from build123d import *

# Parameters (mm, degrees)
F1_DEPTH = 4.7625
F3_D     = 57.15
F4_D     = 25.4


with BuildPart() as f1:
    # F0 (on Front) → F1 (new body, symmetric)
    with BuildSketch(Plane.XZ):
        with BuildLine():
            ThreePointArc((63.5, 161.311665), (-6.276947, 224.500667), (-62.259053, 148.819256))
            ThreePointArc((-62.259053, 148.819256), (0, 161.317577), (62.259053, 148.819256))
            ThreePointArc((62.259053, 148.819256), (63.189002, 155.034718), (63.5, 161.311665))
        make_face()
        with BuildLine():
            ThreePointArc((-62.259053, 148.819256), (-51.584807, 124.281169), (-31.75, 106.319052))
            Line((-31.75, 106.319052), (0, 161.311665))
            Line((0, 161.311665), (31.75, 106.319052))
            ThreePointArc((31.75, 106.319052), (51.584807, 124.281169), (62.259053, 148.819256))
            ThreePointArc((62.259053, 148.819256), (0, 161.317577), (-62.259053, 148.819256))
        make_face()
        with BuildLine():
            ThreePointArc((-107.95, -25.663219), (-84.707387, -48.905833), (-76.2, -80.655833))
            Line((-76.2, -80.655833), (0, -80.655833))
            Line((0, -80.655833), (76.2, -80.655833))
            ThreePointArc((76.2, -80.655833), (84.707387, -48.905833), (107.95, -25.663219))
            Line((107.95, -25.663219), (69.849998, 40.327919))
            Line((69.849998, 40.327919), (31.75, 106.319052))
            ThreePointArc((31.75, 106.319052), (0, 97.811665), (-31.75, 106.319052))
            Line((-31.75, 106.319052), (-69.849998, 40.327919))
            Line((-69.849998, 40.327919), (-107.95, -25.663219))
        make_face()
        with BuildLine():
            Line((69.849998, 40.327919), (107.95, -25.663219))
            ThreePointArc((107.95, -25.663219), (133.423053, -17.466831), (160.010782, -20.491706))
            add(Edge.make_bspline(
                [(69.849998, 40.327919), (69.849999, 40.327918), (86.141954, 12.109423), (123.076369, -4.191142), (160.010782, -20.491706)],
                knots=[108.756574, 108.756574, 108.756574, 108.756574, 108.756578, 217.513155, 217.513155, 217.513155, 217.513155], degree=3))
        make_face()
        with BuildLine():
            ThreePointArc((-160.010782, -20.491706), (-133.423053, -17.466831), (-107.95, -25.663219))
            Line((-107.95, -25.663219), (-69.849998, 40.327919))
            add(Edge.make_bspline(
                [(-160.010782, -20.491706), (-123.076369, -4.191142), (-86.141954, 12.109423), (-69.849999, 40.327918), (-69.849998, 40.327919)],
                knots=[0, 0, 0, 0, 108.756578, 108.756581, 108.756581, 108.756581, 108.756581], degree=3))
        make_face()
        with BuildLine():
            Line((0, 161.311665), (-31.75, 106.319052))
            ThreePointArc((-31.75, 106.319052), (0, 97.811665), (31.75, 106.319052))
            Line((31.75, 106.319052), (0, 161.311665))
        make_face()
        with BuildLine():
            ThreePointArc((160.010782, -20.491706), (139.705119, -80.658788), (97.751729, -128.327549))
            ThreePointArc((97.751729, -128.327549), (165.858505, -138.517587), (203.2, -80.655833))
            ThreePointArc((203.2, -80.655833), (191.284807, -43.625336), (160.010782, -20.491706))
        make_face()
        with BuildLine():
            ThreePointArc((107.95, -25.663219), (84.707387, -48.905833), (76.2, -80.655833))
            Line((76.2, -80.655833), (139.7, -80.655833))
            Line((139.7, -80.655833), (107.95, -25.663219))
        make_face()
        with BuildLine():
            Line((139.7, -80.655833), (76.2, -80.655833))
            ThreePointArc((76.2, -80.655833), (81.838246, -106.814338), (97.751729, -128.327549))
            ThreePointArc((97.751729, -128.327549), (139.705119, -80.658788), (160.010782, -20.491706))
            ThreePointArc((160.010782, -20.491706), (133.423053, -17.466831), (107.95, -25.663219))
            Line((107.95, -25.663219), (139.7, -80.655833))
        make_face()
        with BuildLine():
            Line((31.75, 106.319052), (69.849998, 40.327919))
            add(Edge.make_bspline(
                [(62.259053, 148.819256), (57.908549, 108.682834), (53.558045, 68.546413), (69.849998, 40.327919)],
                knots=[0, 0, 0, 0, 108.756574, 108.756574, 108.756574, 108.756574], degree=3))
            ThreePointArc((62.259053, 148.819256), (51.584807, 124.281169), (31.75, 106.319052))
        make_face()
        with BuildLine():
            Line((0, -80.655833), (-76.2, -80.655833))
            ThreePointArc((-76.2, -80.655833), (-81.838246, -106.814338), (-97.751729, -128.327549))
            add(Edge.make_bspline(
                [(-97.751729, -128.327549), (-65.16782, -104.491691), (-32.58391, -80.655833), (0, -80.655833)],
                knots=[0, 0, 0, 0, 108.756578, 108.756578, 108.756578, 108.756578], degree=3))
        make_face()
        with BuildLine():
            Line((76.2, -80.655833), (0, -80.655833))
            add(Edge.make_bspline(
                [(0, -80.655833), (32.58391, -80.655833), (65.16782, -104.491691), (97.751729, -128.327549)],
                knots=[108.756578, 108.756578, 108.756578, 108.756578, 217.513155, 217.513155, 217.513155, 217.513155], degree=3))
            ThreePointArc((97.751729, -128.327549), (81.838246, -106.814338), (76.2, -80.655833))
        make_face()
        with BuildLine():
            ThreePointArc((-97.751729, -128.327549), (-81.838246, -106.814338), (-76.2, -80.655833))
            Line((-76.2, -80.655833), (-139.7, -80.655833))
            Line((-139.7, -80.655833), (-107.95, -25.663219))
            ThreePointArc((-107.95, -25.663219), (-133.423053, -17.466831), (-160.010782, -20.491706))
            ThreePointArc((-160.010782, -20.491706), (-139.705119, -80.658788), (-97.751729, -128.327549))
        make_face()
        with BuildLine():
            Line((-139.7, -80.655833), (-76.2, -80.655833))
            ThreePointArc((-76.2, -80.655833), (-84.707387, -48.905833), (-107.95, -25.663219))
            Line((-107.95, -25.663219), (-139.7, -80.655833))
        make_face()
        with BuildLine():
            ThreePointArc((-160.010782, -20.491706), (-194.692613, -112.405833), (-97.751729, -128.327549))
            ThreePointArc((-97.751729, -128.327549), (-139.705119, -80.658788), (-160.010782, -20.491706))
        make_face()
        with BuildLine():
            add(Edge.make_bspline(
                [(-69.849998, 40.327919), (-53.558045, 68.546413), (-57.908549, 108.682834), (-62.259053, 148.819256)],
                knots=[108.756581, 108.756581, 108.756581, 108.756581, 217.513155, 217.513155, 217.513155, 217.513155], degree=3))
            Line((-69.849998, 40.327919), (-31.75, 106.319052))
            ThreePointArc((-31.75, 106.319052), (-51.584807, 124.281169), (-62.259053, 148.819256))
        make_face()
    extrude(amount=F1_DEPTH, both=True)

    # F3 (through all)
    with Locations(Plane.XZ.offset(4.7625)):
        with Locations((-139.7, -80.655833), (139.7, -80.655833), (0, 161.311665)):
            Hole(F3_D / 2)

    # F4 (through all)
    with Locations(Plane.XZ.offset(4.7625)):
        with Locations((0, 0)):
            Hole(F4_D / 2)


solid = f1.part
Geometry check sheet. Reference: the model listing, model coordinates, mm. Round coordinates to 2 decimals unless told otherwise and drop trailing zeros. Write each loop counter-clockwise with the first axis right and the second up, starting at its lowest first coordinate (ties: lowest second). Pieces come first, ordered by that corner, then holes.
Item 1: Section check C-C (y = 3). Give the number of separate pieces and of enclosed holes in the cut face, plus the area to 3 significant figures.
Determined:
separate pieces: 1
enclosed holes: 4
area: 63,500 mm2
Item 2: Material ranges on line 1 along Z through (x, y) = (0, 1.75); line 2 along X through (y, z) = (2, -100); line 3 along X through (y, z) = (3, -106.5), recorded low to high.
Determined:
line 1: z = -80.66 to -12.7, 12.7 to 132.74, 189.89 to 224.81
line 2: x = -200.18 to -160.73, -118.67 to -56.6, 56.6 to 118.67, 160.73 to 200.18
line 3: x = -197.7 to -151.89, -127.51 to -66.89, 66.89 to 127.51, 151.89 to 197.7
Item 3: Section check A-A (z = -74.5). Record the boundary of the cut face in (x, y), plus the area to 3 significant figures.
Determined:
outline: (-202.9, -4.76) - (-167.6, -4.76) - (-167.6, 4.76) - (-202.9, 4.76) - close; (-111.8, -4.76) - (111.8, -4.76) - (111.8, 4.76) - (-111.8, 4.76) - close; (167.6, -4.76) - (202.9, -4.76) - (202.9, 4.76) - (167.6, 4.76) - close
area: 2,800 mm2
Item 4: Mould release check, pull along Z, two halves, no side actions. Record for faces 1 (the face through (63.18, -0.07, 154.95)), 2 (the face through (-166.955, 0.067, -72.073)), 3 (the face through (-195.462, -0.067, -111.034)), 4 (the face through (-3, 4.762, -39)): +Z half, -Z half, draft (parallel to the pull), parting line (faces both ways), or undercut.
Determined:
face 1: undercut
face 2: undercut
face 3: parting line
face 4: draft
Item 5: Go/stop test with flat-tipped pins: pin 1 Ø2 at (x, y) = (4, -2.5) entering from -Z; pin 2 Ø4 at (y, z) = (0, -64) entering from +X; pin 3 Ø1.5 at (y, z) = (2.5, -99.5) entering from -X. Record where each tip stops, or that it passes through.
Determined:
pin 1: stops at z = -80.84
pin 2: stops at x = 201.49
pin 3: stops at x = -200.57
Item 6: Section check B-B (z = 170.5). Record the boundary of the cut face in (x, y).
Determined:
outline: (-62.83, -4.76) - (-27.06, -4.76) - (-27.06, 4.76) - (-62.83, 4.76) - close; (27.06, -4.76) - (62.83, -4.76) - (62.83, 4.76) - (27.06, 4.76) - close
